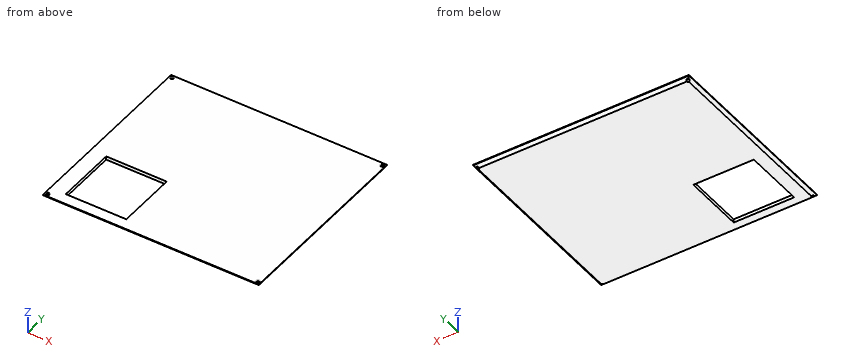
```python
from build123d import *

# Parameters (mm, degrees)
SKETCH1_W           = 157
SKETCH1_H           = 139.5
BOSS_EXTRUDE1_DEPTH = 2.5
CHAMFER1_SIZE       = 2
SKETCH5_W           = 44
SKETCH5_H           = 44
CUT_EXTRUDE1_DEPTH  = 10
SKETCH6_R           = 1
CUT_EXTRUDE2_DEPTH  = 10
FILLET1_R           = 0.5


with BuildPart() as part:
    # Sketch1 → Boss-Extrude1 (new body)
    with BuildSketch(Plane.XY):
        with Locations((78.5, 69.75)):
            Rectangle(SKETCH1_W, SKETCH1_H)
    extrude(amount=BOSS_EXTRUDE1_DEPTH)

    # Chamfer1
    chamfer1_edges = [part.edges().sort_by_distance(p)[0] for p in [
        (78.5, 139.5, 0),
        (157, 69.75, 0),
        (78.5, 0, 0),
        (0, 69.75, 0),
    ]]
    chamfer(chamfer1_edges, length=CHAMFER1_SIZE)

    # Sketch5 → Cut-Extrude1 (cut)
    with BuildSketch(Plane(origin=(0, 0, 0), x_dir=(-1, 0, 0), z_dir=(0, 0, -1))):
        with Locations((-33.223972079, 30)):
            Rectangle(SKETCH5_W, SKETCH5_H)
    extrude(amount=-CUT_EXTRUDE1_DEPTH, mode=Mode.SUBTRACT)

    # Sketch6 → Cut-Extrude2 (cut)
    with BuildSketch(Plane.XY.offset(2.5)):
        with Locations((155, 137.5)):
            Circle(SKETCH6_R)
        with Locations((2, 137.5)):
            Circle(SKETCH6_R)
        with Locations((155, 2)):
            Circle(SKETCH6_R)
        with Locations((2, 2)):
            Circle(SKETCH6_R)
    extrude(amount=-CUT_EXTRUDE2_DEPTH, mode=Mode.SUBTRACT)

    # Fillet1
    fillet1_edges = [part.edges().sort_by_distance(p)[0] for p in [
        (154, 2, 2.5),
        (154, 137.5, 2.5),
        (1, 137.5, 2.5),
        (1, 2, 2.5),
    ]]
    fillet(fillet1_edges, radius=FILLET1_R)


solid = part.part
```
Model file for the job. Use its own axes, mm. Coordinates: 2 decimals unless noted, no trailing zeros. Order: outer loops, then holes, each group sorted by start corner. A loop starts at its lowest first (then second) coordinate and runs counter-clockwise, first axis right, second up. Notation, with made-up numbers: (63, 60) - (90, 60) arc R28 ccw to (90, 89) - close; hole circle Ø3 at (9.25, 69). An arc over 180 degrees is marked (long way). Return JSON: item names as keys, results as strings. Group by question number.
1) Saw through at A-A, the plane x = 28.5. Write the cut outline in (y, z).
2) Saw through at B-B, the plane z = 1.45. Write the cut outline in (x, y).
3) Probe line 1 (Y direction, x = 17, z = 2); line 2 (Y direction, x = 155, z = 1.4); line 3 (Y direction, x = 2, z = 1.25). List the from-to ranges inside material, lowest first. Write a range as from..to.
4) Flat gauge pin, fed straight in: P1, Ø1.6, axis at x = 2, y = 137.5, coming from the -Z side. Where does the tip first touch, or does it go through?
Values found:
{
 "1": {"outline": "(0, 2) - (2, 0) - (8, 0) - (8, 2.5) - (0, 2.5) - close; (52, 0) - (137.5, 0) - (139.5, 2) - (139.5, 2.5) - (52, 2.5) - close"},
 "2": {"outline": "(0.55, 0.55) - (156.45, 0.55) - (156.45, 138.95) - (0.55, 138.95) - close; hole circle Ø2 at (2, 2); hole circle Ø2 at (2, 137.5); hole (11.22, 8) - (55.22, 8) - (55.22, 52) - (11.22, 52) - close; hole circle Ø2 at (155, 2); hole circle Ø2 at (155, 137.5)"},
 "3": {"line 1": "y = 0..8, 52..139.5", "line 2": "y = 0.6..1, 3..136.5, 138.5..138.9", "line 3": "y = 0.75..1, 3..136.5, 138.5..138.75"},
 "4": {"P1": "passes through"}
}
